CAD build for the part. Positions are in the model's coordinates, mm. Face numbers are marked on the shaded views. A direction names the side the tool comes from. Give positions to 0.01 mm unless a question says otherwise; leave off trailing zeros. Loops run counter-clockwise (first coordinate to the right, second up) from the corner with the lowest first, then second, coordinate; pieces in that order, holes last. Notation, with made-up numbers: M 33.25,81 L 60.25,81 A20 cw 60.25,97 Z; hole C -33,5 d11. An arc over 180 degrees is marked long. Answer as CSV lines item,"result".
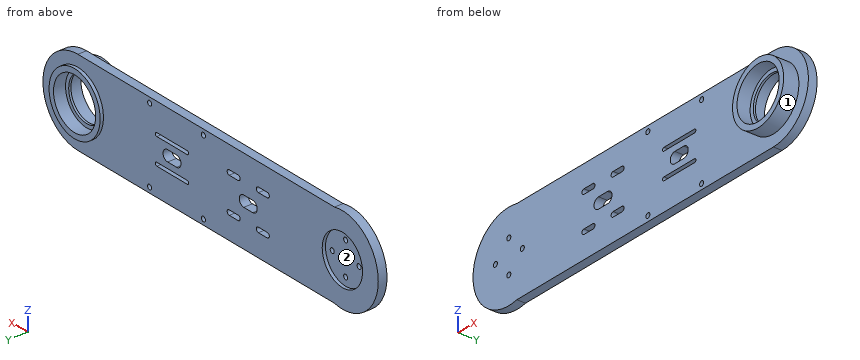
```python
from build123d import *

# Parameters (mm, degrees)
SKETCH4_R                = 22.5
SKETCH4_R_2              = 2.25
BOSS_EXTRUDE3_DEPTH      = 5
SKETCH4_4_R              = 28.5
SKETCH4_4_R_2            = 22.5
BOSS_EXTRUDE4_DEPTH      = 8
SKETCH4_5_R              = 28.5
SKETCH4_5_R_2            = 23.5
BOSS_EXTRUDE5_DEPTH      = 11
BOSS_EXTRUDE5_DEPTH_BACK = 14
SKETCH4_6_R              = 23.5
SKETCH4_6_R_2            = 20
BOSS_EXTRUDE6_DEPTH      = 2
SKETCH5_R                = 2.25
CUT_EXTRUDE1_DEPTH       = 10


with BuildPart() as part:
    # Sketch4 → Boss-Extrude3 (new body)
    with BuildSketch(Plane(origin=(0, 0, 0), x_dir=(1, 0, 0), z_dir=(0, 1, 0))):
        Circle(SKETCH4_R)
        with Locations((0, -15)):
            Circle(SKETCH4_R_2, mode=Mode.SUBTRACT)
        with Locations((-15, 0)):
            Circle(SKETCH4_R_2, mode=Mode.SUBTRACT)
        with Locations((0, 15)):
            Circle(SKETCH4_R_2, mode=Mode.SUBTRACT)
        with Locations((15, 0)):
            Circle(SKETCH4_R_2, mode=Mode.SUBTRACT)
    extrude(amount=BOSS_EXTRUDE3_DEPTH)

    # Sketch4_4 → Boss-Extrude4 (add)
    with BuildSketch(Plane(origin=(0, 0, 0), x_dir=(1, 0, 0), z_dir=(0, 1, 0))):
        with BuildLine():
            ThreePointArc((8.888194417, 39), (-40, 0), (8.888194417, -39))
            Line((8.888194417, -39), (295, -39))
            ThreePointArc((295, -39), (334, 0), (295, 39))
            Line((295, 39), (8.888194417, 39))
        make_face()
        with BuildLine():
            Line((93.736544033, -18.513455967), (83.736544033, -18.513455967))
            ThreePointArc((83.736544033, -18.513455967), (81.486544033, -16.263455967), (83.736544033, -14.013455967))
            Line((83.736544033, -14.013455967), (93.736544033, -14.013455967))
            ThreePointArc((93.736544033, -14.013455967), (95.986544033, -16.263455967), (93.736544033, -18.513455967))
        make_face(mode=Mode.SUBTRACT)
        with BuildLine():
            Line((126.263455967, -18.513455967), (116.263455967, -18.513455967))
            ThreePointArc((116.263455967, -18.513455967), (114.013455967, -16.263455967), (116.263455967, -14.013455967))
            Line((116.263455967, -14.013455967), (126.263455967, -14.013455967))
            ThreePointArc((126.263455967, -14.013455967), (128.513455967, -16.263455967), (126.263455967, -18.513455967))
        make_face(mode=Mode.SUBTRACT)
        with BuildLine():
            Line((172.97918472, -10.42081528), (207.02081528, -10.42081528))
            ThreePointArc((207.02081528, -10.42081528), (208.62081528, -12.02081528), (207.02081528, -13.62081528))
            Line((207.02081528, -13.62081528), (172.97918472, -13.62081528))
            ThreePointArc((172.97918472, -13.62081528), (171.37918472, -12.02081528), (172.97918472, -10.42081528))
        make_face(mode=Mode.SUBTRACT)
        with BuildLine():
            ThreePointArc((100, -5), (95, 0), (100, 5))
            Line((100, 5), (110, 5))
            ThreePointArc((110, 5), (115, 0), (110, -5))
            Line((110, -5), (100, -5))
        make_face(mode=Mode.SUBTRACT)
        with BuildLine():
            ThreePointArc((83.736544033, 14.013455967), (81.486544033, 16.263455967), (83.736544033, 18.513455967))
            Line((83.736544033, 18.513455967), (93.736544033, 18.513455967))
            ThreePointArc((93.736544033, 18.513455967), (95.986544033, 16.263455967), (93.736544033, 14.013455967))
            Line((93.736544033, 14.013455967), (83.736544033, 14.013455967))
        make_face(mode=Mode.SUBTRACT)
        with BuildLine():
            ThreePointArc((116.263455967, 14.013455967), (114.013455967, 16.263455967), (116.263455967, 18.513455967))
            Line((116.263455967, 18.513455967), (126.263455967, 18.513455967))
            ThreePointArc((126.263455967, 18.513455967), (128.513455967, 16.263455967), (126.263455967, 14.013455967))
            Line((126.263455967, 14.013455967), (116.263455967, 14.013455967))
        make_face(mode=Mode.SUBTRACT)
        with BuildLine():
            ThreePointArc((195, 5), (200, 0), (195, -5))
            Line((195, -5), (185, -5))
            ThreePointArc((185, -5), (180, 0), (185, 5))
            Line((185, 5), (195, 5))
        make_face(mode=Mode.SUBTRACT)
        with BuildLine():
            ThreePointArc((207.02081528, 13.62081528), (208.62081528, 12.02081528), (207.02081528, 10.42081528))
            Line((207.02081528, 10.42081528), (172.97918472, 10.42081528))
            ThreePointArc((172.97918472, 10.42081528), (171.37918472, 12.02081528), (172.97918472, 13.62081528))
            Line((172.97918472, 13.62081528), (207.02081528, 13.62081528))
        make_face(mode=Mode.SUBTRACT)
        with Locations((295, 0)):
            Circle(SKETCH4_4_R, mode=Mode.SUBTRACT)
        Circle(SKETCH4_4_R_2, mode=Mode.SUBTRACT)
    extrude(amount=BOSS_EXTRUDE4_DEPTH)

    # Sketch4_5 → Boss-Extrude5 (add, two sides)
    with BuildSketch(Plane(origin=(0, 0, 0), x_dir=(1, 0, 0), z_dir=(0, 1, 0))) as boss_extrude5_sk:
        with Locations((295, 0)):
            Circle(SKETCH4_5_R)
        with Locations((295, 0)):
            Circle(SKETCH4_5_R_2, mode=Mode.SUBTRACT)
    extrude(amount=BOSS_EXTRUDE5_DEPTH)
    extrude(boss_extrude5_sk.sketch, amount=-BOSS_EXTRUDE5_DEPTH_BACK)

    # Sketch4_6 → Boss-Extrude6 (add)
    with BuildSketch(Plane(origin=(0, 0, 0), x_dir=(1, 0, 0), z_dir=(0, 1, 0))):
        with Locations((295, 0)):
            Circle(SKETCH4_6_R)
        with Locations((295, 0)):
            Circle(SKETCH4_6_R_2, mode=Mode.SUBTRACT)
    extrude(amount=-BOSS_EXTRUDE6_DEPTH)

    # Sketch5 → Cut-Extrude1 (cut)
    with BuildSketch(Plane.XZ):
        with Locations((155, 34)):
            Circle(SKETCH5_R)
        with Locations((215, 34)):
            Circle(SKETCH5_R)
        with Locations((215, -34)):
            Circle(SKETCH5_R)
        with Locations((155, -34)):
            Circle(SKETCH5_R)
    extrude(amount=-CUT_EXTRUDE1_DEPTH, mode=Mode.SUBTRACT)


solid = part.part
```
Q1. Cut at C-C (x = 41.5). Write the cut outline in (y, z), and give its area (3 significant figures).
Solution:
outline,"M 0,-39 L 8,-39 L 8,39 L 0,39 Z"
area,"624 mm²"
Q2. Cut at A-A (y = -9). Write the cut outline in (x, z).
Solution:
outline,"C 295,0 d57; hole C 295,0 d47"
Q3. Cut at B-B (x = -7). Write the cut outline in (y, z), and give its area (3 significant figures).
Solution:
outline,"M 0,-39.38 L 8,-39.38 L 8,-21.38 L 5,-21.38 L 5,21.38 L 8,21.38 L 8,39.38 L 0,39.38 Z"
area,"502 mm²"
Q4. Which spindle directions (+Z, -Z, +X, -X, +Y, -Y) get a long thin tool onto all of the face, cutting with end or side? Do the marked faces 1 and 2. Say none if no direction does.
Solution:
face 1,"-Y"
face 2,"+Y"
Q5. Wall check: line 1 (Z direction, x = 0, y = 3.6); line 2 (Z direction, x = 15, y = 2); line 3 (Z direction, x = 215, y = 3.25). Give the ranges that are in metal, low to high. Write a range as [from, to].
Solution:
line 1,"z = [-40, -17.25], [-12.75, 12.75], [17.25, 40]"
line 2,"z = [-39, -2.25], [2.25, 39]"
line 3,"z = [-39, -36.25], [-31.75, 31.75], [36.25, 39]"
Q6. Pin check, flat tips, straight feed: P1, Ø6.5, axis at x = 197.5, y = 2.5, coming from the +Z side; P2, Ø2.5, axis at x = 90, y = 3, coming from the -Z side; P3, Ø6, axis at x = 0, z = 15, coming from the -Y side. Stop position of each tip, or through.
Solution:
P1,"stops at z = 39"
P2,"stops at z = -39"
P3,"stops at y = 0"
